from build123d import *

# Parameters (mm, degrees)
SKETCH_1_R          = 3
SKETCH_1_W          = 90
SKETCH_1_H          = 120
SKETCH_1_R_2        = 10
SKETCH_1_R_3        = 7.5
EXTRUDE_2_DEPTH     = 3
EXTRUDE_START       = -3
SKETCH_2_R          = 10
SKETCH_2_R_2        = 7.5
EXTRUDE_3_DEPTH     = 3
CUT_EXTRUDE_START   = -3
SKETCH_3_R          = 3
SKETCH_3_W          = 90
SKETCH_3_H          = 120
CUT_EXTRUDE_2_DEPTH = 3
SKETCH_4_W          = 10
SKETCH_4_H          = 50
EXTRUDE_4_DEPTH     = 30
SKETCH_5_R          = 8
CUT_EXTRUDE_3_DEPTH = 30
SKETCH_6_R          = 2.6
CUT_EXTRUDE_5_DEPTH = 10


with BuildPart() as part:
    # 草图1 → 凸台-拉伸2 (new body)
    # profile 1 of 9: a face of its own
    with BuildSketch(Plane.XY):
        Polygon((195, -115), (195, 115), (190, 115), (190, 120), (115, 120), (115, 75), (75, 75), (-90, 75), (-130, 75), (-130, 120), (-175, 120), (-175, 90), (-195, 90), (-195, -90), (-175, -90), (-175, -120), (-130, -120), (-130, -75), (-90, -75), (75, -75), (115, -75), (115, -120), (190, -120), (190, -115), align=None)
        with Locations((-184.089468205, -70)):
            Circle(SKETCH_1_R, mode=Mode.SUBTRACT)
        with Locations((-87, -69)):
            Circle(SKETCH_1_R, mode=Mode.SUBTRACT)
        with Locations((-184.089468205, 70)):
            Circle(SKETCH_1_R, mode=Mode.SUBTRACT)
        with Locations((-87, 69)):
            Circle(SKETCH_1_R, mode=Mode.SUBTRACT)
        Rectangle(SKETCH_1_W, SKETCH_1_H, mode=Mode.SUBTRACT)
        with Locations((75, 0)):
            Circle(SKETCH_1_R_2, mode=Mode.SUBTRACT)
        with Locations((117.5, 0)):
            Circle(SKETCH_1_R_3, mode=Mode.SUBTRACT)
    # profile 2 of 9: a face of its own
    with BuildSketch(Plane.XY):
        Polygon((-130, 120), (-90, 75), (-130, 75), align=None)
    # profile 3 of 9: a face of its own
    with BuildSketch(Plane.XY):
        Polygon((-175, 120), (-175, 90), (-195, 90), align=None)
    # profile 4 of 9: a face of its own
    with BuildSketch(Plane.XY):
        Polygon((-175, -120), (-195, -90), (-175, -90), align=None)
    # profile 5 of 9: a face of its own
    with BuildSketch(Plane.XY):
        Polygon((-130, -120), (-130, -75), (-90, -75), align=None)
    # profile 6 of 9: a face of its own
    with BuildSketch(Plane.XY):
        Polygon((115, -120), (75, -75), (115, -75), align=None)
        with Locations((104.379549532, -93)):
            Circle(SKETCH_1_R, mode=Mode.SUBTRACT)
    # profile 7 of 9: a face of its own
    with BuildSketch(Plane.XY):
        Polygon((115, 120), (115, 75), (75, 75), align=None)
        with Locations((104.379549532, 93)):
            Circle(SKETCH_1_R, mode=Mode.SUBTRACT)
    # profile 8 of 9: a face of its own
    with BuildSketch(Plane.XY):
        Polygon((190, 120), (195, 115), (190, 115), align=None)
    # profile 9 of 9: a face of its own
    with BuildSketch(Plane.XY):
        Polygon((190, -115), (190, -120), (195, -115), align=None)
    extrude(amount=EXTRUDE_2_DEPTH)

    # 草图2 → 凸台-拉伸3 (add)
    with BuildSketch(Plane.XY.offset(3).offset(EXTRUDE_START)):
        with Locations((75, 0)):
            Circle(SKETCH_2_R)
        with Locations((117.5, 0)):
            Circle(SKETCH_2_R_2)
    extrude(amount=EXTRUDE_3_DEPTH)

    # 草图3 → 切除-拉伸2 (cut)
    # profile 1 of 3: a face of its own
    with BuildSketch(Plane.XY.offset(3).offset(CUT_EXTRUDE_START)):
        Polygon((115, 120), (115, -120), (75, -75), (-90, -75), (-130, -120), (-175, -120), (-195, -90), (-195, 90), (-175, 120), (-130, 120), (-90, 75), (75, 75), align=None)
        with Locations((-184.089468205, -70)):
            Circle(SKETCH_3_R, mode=Mode.SUBTRACT)
        with Locations((-87, 69)):
            Circle(SKETCH_3_R, mode=Mode.SUBTRACT)
        with Locations((104.379549532, 93)):
            Circle(SKETCH_3_R, mode=Mode.SUBTRACT)
        with Locations((104.379549532, -93)):
            Circle(SKETCH_3_R, mode=Mode.SUBTRACT)
        with Locations((-87, -69)):
            Circle(SKETCH_3_R, mode=Mode.SUBTRACT)
        with Locations((-184.089468205, 70)):
            Circle(SKETCH_3_R, mode=Mode.SUBTRACT)
        Rectangle(SKETCH_3_W, SKETCH_3_H, mode=Mode.SUBTRACT)
    # profile 2 of 3: a face of its own
    with BuildSketch(Plane.XY.offset(3).offset(CUT_EXTRUDE_START)):
        Polygon((120, -120), (115, -115), (115, -120), align=None)
    # profile 3 of 3: a face of its own
    with BuildSketch(Plane.XY.offset(3).offset(CUT_EXTRUDE_START)):
        Polygon((120, 120), (115, 120), (115, 115), align=None)
    extrude(amount=CUT_EXTRUDE_2_DEPTH, mode=Mode.SUBTRACT)

    # 草图4 → 凸台-拉伸4 (add)
    with BuildSketch(Plane.XY.offset(3)):
        with Locations((120, 0)):
            Rectangle(SKETCH_4_W, SKETCH_4_H)
    extrude(amount=EXTRUDE_4_DEPTH)

    # 草图5 → 切除-拉伸3 (cut)
    with BuildSketch(Plane.ZY.offset(-115)):
        with Locations(Location((18, 0, 0), (0, 0, 270))):
            Circle(SKETCH_5_R)
    extrude(amount=-CUT_EXTRUDE_3_DEPTH, mode=Mode.SUBTRACT)

    # 草图6 → 切除-拉伸5 (cut)
    with BuildSketch(Plane.XY.offset(3)):
        with Locations((150, 90)):
            Circle(SKETCH_6_R)
        with Locations((180, 90)):
            Circle(SKETCH_6_R)
        with Locations((180, 110)):
            Circle(SKETCH_6_R)
        with Locations((150, 110)):
            Circle(SKETCH_6_R)
        with Locations((150, -90)):
            Circle(SKETCH_6_R)
        with Locations((150, -110)):
            Circle(SKETCH_6_R)
        with Locations((180, -110)):
            Circle(SKETCH_6_R)
        with Locations((180, -90)):
            Circle(SKETCH_6_R)
    extrude(amount=-CUT_EXTRUDE_5_DEPTH, mode=Mode.SUBTRACT)


solid = part.part
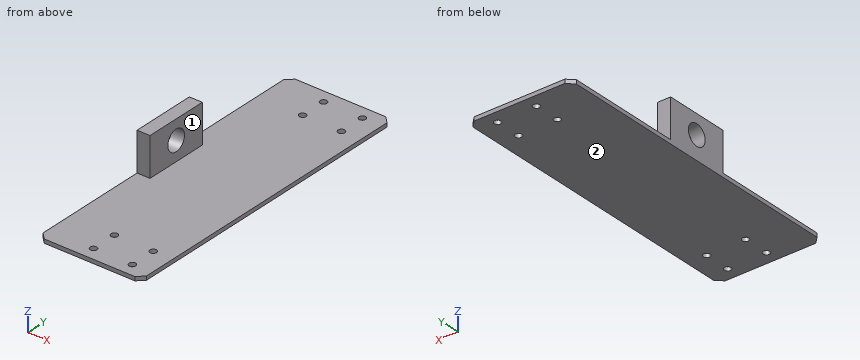
Verification items for the finished model (mm, model axes). Face numbers are marked on the shaded views. A direction names the side the tool comes from. Give positions to 0.01 mm unless a question says otherwise; leave off trailing zeros. Loops run counter-clockwise (first coordinate to the right, second up) from the corner with the lowest first, then second, coordinate; pieces in that order, holes last. Notation, with made-up numbers: (25.5, 45) - (77.5, 45) arc R21 ccw to (77.5, 61) - close; hole circle Ø9 at (-7.5, -21.75). An arc over 180 degrees is marked (long way). Write item = value, one per line. Start each with the question number.
Q1. Cross-section at D-D, the plane y = 110. Enter the section's corners in (x, z), and give its area (3 significant figures).
Q2. Tool access check on the marked faces 1 and 2. Record the directions out of +Z, -Z, +X, -X, +Y, -Y that give a thin tool (end or side, any length) a straight path to the whole face; none if there is none.
Q3. Thickness scan on line 1 (Y direction, x = 180, z = 1); line 2 (Z direction, x = 135.5, y = -19); line 3 (X direction, y = -18, z = 11.5). Record the ranges inside material, lowest first.
Q4. Depth check by flat-ended pin: P1, Ø11, axis at x = 119.5, z = 16, coming from the -Y side; P2, Ø5, axis at x = 174, y = -3, coming from the +Z side; P3, Ø11, axis at x = 118, z = 16.5, coming from the +Y side. Enter the tip coordinate at first touch or a pass-through.
Q5. Cross-section at C-C, the plane x = 180. Enter the section's corners in (y, z).
Q6. Cross-section at A-A, the plane y = 0. Enter the section's corners in (x, z), and give its area (3 significant figures).
Q7. Cross-section at B-B, the plane z = 18. Enter the section's corners in (x, y).
Answer key:
q1.outline = (115, 0) - (147.4, 0) - (147.4, 3) - (115, 3) - close; (152.6, 0) - (177.4, 0) - (177.4, 3) - (152.6, 3) - close; (182.6, 0) - (195, 0) - (195, 3) - (182.6, 3) - close
q1.area = 209 mm^2
q2.face_1 = +Z, +X, +Y, -Y
q2.face_2 = -Z, +X, -X, +Y, -Y
q3.line_1 = -120 to -112.6, -107.4 to -92.6, -87.4 to 87.4, 92.6 to 107.4, 112.6 to 120
q3.line_2 = 0 to 3
q3.line_3 = 115 to 125
q4.P1 = -25
q4.P2 = 3
q4.P3 = 25
q5.outline = (-120, 0) - (-112.6, 0) - (-112.6, 3) - (-120, 3) - close; (-107.4, 0) - (-92.6, 0) - (-92.6, 3) - (-107.4, 3) - close; (-87.4, 0) - (87.4, 0) - (87.4, 3) - (-87.4, 3) - close; (92.6, 0) - (107.4, 0) - (107.4, 3) - (92.6, 3) - close; (112.6, 0) - (120, 0) - (120, 3) - (112.6, 3) - close
q6.outline = (115, 0) - (195, 0) - (195, 3) - (125, 3) - (125, 10) - (115, 10) - close; (115, 26) - (125, 26) - (125, 33) - (115, 33) - close
q6.area = 380 mm^2
q7.outline = (115, -25) - (125, -25) - (125, -8) - (115, -8) - close; (115, 8) - (125, 8) - (125, 25) - (115, 25) - close
